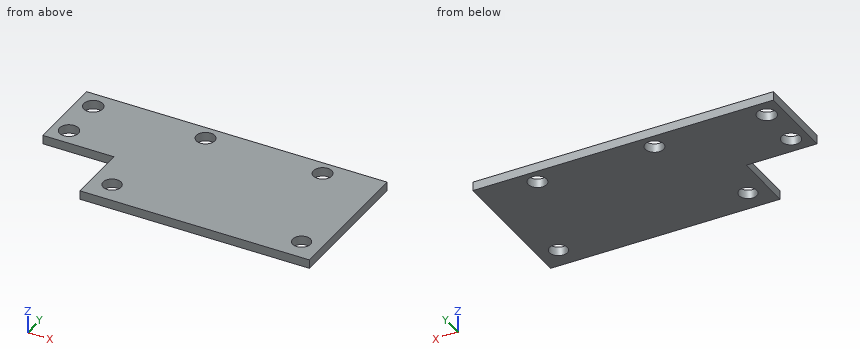
Autodesk Inventor part; units mm, degrees
ref_plane "YZ Plane" through (0, 0, 0) normal (1, 0, 0) x (0, 1, 0)
ref_plane "XZ Plane" through (0, 0, 0) normal (0, 1, 0) x (-1, 0, 0)
ref_plane "XY Plane" through (0, 0, 0) normal (0, 0, 1) x (1, 0, 0)
sketch "Sketch1" plane through (0, 0, 0) normal (0, 0, 1) x (1, 0, 0)
  line L0 (0, 0) -> (-56.9976, 0)
  line L1 (-56.9976, 50.8) -> (0, 50.8)
  line L2 (0, 50.8) -> (-7.493, 50.8)
  line L3 (-7.493, 50.8) -> (-7.493, 44.45)
  line L4 (-56.9976, 50.8) -> (-49.5046, 50.8)
  line L5 (-49.5046, 50.8) -> (-49.5046, 44.45)
  line L6 (-56.9976, 50.8) -> (-69.6976, 50.8)
  line L7 (-69.6976, 50.8) -> (-69.6976, 0)
  line L8 (-69.6976, 0) -> (-56.9976, 0)
  line L9 (0, 50.8) -> (8.89, 50.8)
  line L10 (8.89, 0) -> (0, 0)
  line L11 (0, 50.8) -> (12.7, 50.8)
  line L12 (12.7, 50.8) -> (12.7, 0)
  line L13 (12.7, 0) -> (0, 0)
  dimension "d1" = 56.9976
  dimension "d2" = 50.8
  dimension "d3" = 7.493
  dimension "d4" = 6.35
  dimension "d5" = 7.493
  dimension "d19" = 6.35
  dimension "d48" = 12.7
  dimension "d51" = 50.8
  dimension "d57" = 12.7
extrude "Plate5" add sketch "Sketch1" along normal blind 3.175
sketch "Sketch6" plane through (0, 0, 3.175) normal (0, 0, 1) x (1, 0, 0)
  circle A0 centre (-7.488, 45.44) radius 3.3
  circle A1 centre (-49.488, 45.44) radius 3.3
  point P0 (0, 0)
extrude "Cut1" cut sketch "Sketch6" against normal blind 3.175
sketch "Sketch7" plane through (12.7, 0, 0) normal (1, 0, 0) x (0, 0, -1)
  line L0 (-3.175, 50.8) -> (-3.175, 0)
  line L1 (0, 0) -> (-3.175, 0)
  line L2 (0, 0) -> (0, 50.8)
  line L3 (0, 50.8) -> (-3.175, 50.8)
sketch "Sketch8" plane through (0, 0, 0) normal (0, 0, -1) x (-1, 0, 0)
  circle A0 centre (-5.5012, 7.9858) radius 3.2
  circle A1 centre (62.4988, 7.9858) radius 3.2
  point P0 (0, 0)
extrude "Cut2" cut sketch "Sketch8" against normal blind 3.175
sketch "Sketch12" plane through (-69.6976, 0, 0) normal (-1, 0, 0) x (0, 0, 1)
  line L0 (3.175, 0) -> (3.175, 50.8)
  line L1 (0, 50.8) -> (3.175, 50.8)
  line L2 (0, 50.8) -> (0, 0)
  line L3 (0, 0) -> (3.175, 0)
extrude "Extrusion3" add sketch "Sketch12" along normal blind 25.4
sketch "Sketch10" plane through (0, 0, 0) normal (0, 0, -1) x (-1, 0, 0)
  line L0 (69.6976, 0) -> (-12.7, 0)
  line L1 (107.7976, 22.225) -> (69.6976, 22.225)
  line L2 (69.6976, 22.225) -> (69.6976, 0)
  circle A0 centre (89.254, 44.45) radius 3.3782
  circle A1 centre (89.254, 28.575) radius 3.3782
  line L3 (69.6976, 0) -> (95.0976, 0)
  line L4 (95.0976, 0) -> (95.0976, 22.225)
  point P0 (0, 0)
  dimension "d67" = 38.1
  dimension "d72" = 25.4
extrude "Extrusion4" cut sketch "Sketch10" against normal blind 25.4
equation "\"d60\" = Thickness"
equation "\"d62\" = Thickness"
equation "\"BendRadius\" = Thickness"
equation "\"BendReliefWidth\" = Thickness"
equation "\"BendReliefDepth\" = 0.5 * Thickness"
equation "\"CornerReliefSize\" = 4 * Thickness"
equation "\"MinimumRemnant\" = 2 * Thickness"
equation "\"TransitionRadius\" = BendRadius"
equation "\"JacobiRadiusSize\" = BendRadius"
equation "\"GapSize\" = Thickness"
equation "\"d8\" = BendRadius"
equation "\"d56\" = BendRadius"
properties part number "face mount" material "Aluminum 6061"
Could you check a few things on this model? Use its own coordinates, in mm. Give positions to 0.01 mm unless a question says otherwise; leave off trailing zeros. Loops run counter-clockwise (first coordinate to the right, second up) from the corner with the lowest first, then second, coordinate; pieces in that order, holes last. Notation, with made-up numbers: M 14.25,86.5 L 54.25,86.5 A32 cw 54.25,115.5 Z; hole C 40.5,80.5 d9. An arc over 180 degrees is marked long. Answer as a JSON object with one key per item and string values.
Q1. For P1, Ø1, axis at x = -84.5, z = 1.5, coming from the -Y side (3 decimals), with a flat end and sliding along its axis, tell me the tip position at first contact or that it passes through.
Values found:
{"P1": "stops at y = 22.225"}
Q2. Suppose I cut it at B-B, the plane z = 1.55. List the corners of the cut face in (x, y) for me (3 decimals).
Values found:
{"outline": "M -95.098,22.225 L -69.698,22.225 L -69.698,0 L 12.7,0 L 12.7,50.8 L -95.098,50.8 Z; hole C -89.254,28.575 d6.756; hole C -89.254,44.45 d6.756; hole C -62.499,7.986 d6.4; hole C -49.488,45.44 d6.6; hole C -7.488,45.44 d6.6; hole C 5.501,7.986 d6.4"}
Q3. Suppose I cut it at C-C, the plane x = 4. List the corners of the cut face in (y, z) for me (3 decimals), plus the area to 3 significant figures.
Values found:
{"outline": "M 0,0 L 5.16,0 L 5.16,3.175 L 0,3.175 Z; M 10.812,0 L 50.8,0 L 50.8,3.175 L 10.812,3.175 Z", "area": "143 mm²"}
Q4. Suppose I cut it at D-D, the plane y = 46.5. List the corners of the cut face in (x, z) for me (3 decimals), plus the area to 3 significant figures.
Values found:
{"outline": "M -95.098,0 L -91.939,0 L -91.939,3.175 L -95.098,3.175 Z; M -86.569,0 L -52.613,0 L -52.613,3.175 L -86.569,3.175 Z; M -46.363,0 L -10.613,0 L -10.613,3.175 L -46.363,3.175 Z; M -4.363,0 L 12.7,0 L 12.7,3.175 L -4.363,3.175 Z", "area": "286 mm²"}
Q5. If I drill on probe 1 along X at (y, z) = (45, 2.6); probe 2 along Y at (x, z) = (-90, 1.2) (3 decimals); probe 3 along Y at (x, z) = (-85, 2.5) (3 decimals), over which ranges is the centre line in solid material (lowest first)? Write a range as [from, to].
Values found:
{"probe 1": "x = [-95.1, -92.59], [-85.92, -52.76], [-46.22, -10.76], [-4.22, 12.7]", "probe 2": "y = [22.225, 25.28], [31.87, 41.155], [47.745, 50.8]", "probe 3": "y = [22.225, 50.8]"}
Q6. Suppose I cut it at A-A, the plane y = 6. List the corners of the cut face in (x, z) for me (1 decimal), plus the area to 3 significant figures.
Values found:
{"outline": "M -69.7,0 L -65,0 L -65,3.2 L -69.7,3.2 Z; M -60,0 L 3,0 L 3,3.2 L -60,3.2 Z; M 8,0 L 12.7,0 L 12.7,3.2 L 8,3.2 Z", "area": "230 mm²"}
